Read the model definition and answer for the solid it produces. Units are mm, in the model's axes. A direction names the side the tool comes from. Give positions to 0.01 mm unless a question says otherwise; leave off trailing zeros. Loops run counter-clockwise (first coordinate to the right, second up) from the corner with the lowest first, then second, coordinate; pieces in that order, holes last.
(1) Find section B-B, the plane y = 40. Write down the section's boundary in (x, z), then the cut area to 3 significant figures.
(2) Each of these flat-tipped pins is pushed along its axis until it touches: P1, Ø19, axis at y = 73.5, z = -20, coming from the -X side; P2, Ø3, axis at x = 30, y = 67, coming from the +Z side; P3, Ø3, axis at x = 30.5, z = 5.5, coming from the +Y side. Where does it stop, or does it pass through?
(3) Which of the six approach directions +Z, -Z, +X, -X, +Y, -Y give full straight-line access (tool end or side, diameter ignored) to faces 4 (the face through (56, 12.5, -15)), 5 (the face through (3.89, 43.24, 5.27)), 6 (the face through (13.05, 23.01, 6.51))?
(4) Find section A-A, the plane x = 30. State how many separate pieces and enclosed holes the cut face has, then the cut area to 3 significant figures.
(5) Determine the mould class of faces 1 (the face through (30, 80, -3)), 2 (the face through (4, 4, -30)), 3 (the face through (3.5, 65, -2.5)) for opening direction Y: pulls with the +Y half, pulls with the -Y half, needs draft (parallel to the pull), parting line crosses it, or undercut.
(6) Find section D-D, the plane z = -17. Write down the section's boundary in (x, y).
(7) Straight lines are drawn through the part: probe 1 along Y at (x, z) = (56, -23); probe 2 along Z at (x, y) = (55.75, 5); probe 3 along Y at (x, z) = (52, -4.5). For each, find the intervals that lie inside material, in ascending order.
```python
from build123d import *

# Parameters (mm, degrees)
SKETCH1_W               = 60
SKETCH1_H               = 80
BOSS_EXTRUDE1_DEPTH     = 7
SKETCH2_W               = 7
SKETCH2_H               = 12.5
BOSS_EXTRUDE2_DEPTH     = 30
SKETCH3_R               = 2.6
CUT_EXTRUDE1_DEPTH      = 50
SKETCH4_R               = 25
CUT_EXTRUDE2_DEPTH      = 107.625512894
SKETCH6_R               = 2.1
CUT_EXTRUDE3_DEPTH      = 107.625512894
MIRROR2_COPY_1_SKETCH_W = 7
MIRROR2_COPY_1_SKETCH_H = 12.5
MIRROR2_COPY_1_DEPTH    = 30
MIRROR2_COPY_2_SKETCH_R = 2.6
MIRROR2_COPY_2_DEPTH    = 50
CHAMFER1_SIZE           = 5
CHAMFER2_SIZE           = 5
SKETCH9_W               = 46
SKETCH9_H               = 7.5
BOSS_EXTRUDE4_DEPTH     = 5
CHAMFER3_SIZE           = 5
SKETCH20_R              = 25
SKETCH20_R_2            = 23
BOSS_EXTRUDE5_DEPTH     = 1
CUT_EXTRUDE5_DEPTH      = 3.5


with BuildPart() as part:
    # Sketch1 → Boss-Extrude1 (new body)
    with BuildSketch(Plane.XY):
        with Locations((30, 40)):
            Rectangle(SKETCH1_W, SKETCH1_H)
    extrude(amount=BOSS_EXTRUDE1_DEPTH)

    # Sketch2 → Boss-Extrude2 (add)
    with BuildSketch(Plane(origin=(0, 0, 0), x_dir=(-1, 0, 0), z_dir=(0, 0, -1))):
        with Locations((-3.5, 73.75)):
            Rectangle(SKETCH2_W, SKETCH2_H)
    boss_extrude2 = extrude(amount=BOSS_EXTRUDE2_DEPTH)

    # Sketch3 → Cut-Extrude1 (cut)
    with BuildSketch(Plane.ZY):
        with Locations((-13, 75)):
            Circle(SKETCH3_R)
        with Locations((-23, 75)):
            Circle(SKETCH3_R)
    cut_extrude1 = extrude(amount=-CUT_EXTRUDE1_DEPTH, mode=Mode.SUBTRACT)

    # Sketch4 → Cut-Extrude2 (cut, through all)
    with BuildSketch(Plane.XY.offset(7)):
        with Locations((30, 40)):
            Circle(SKETCH4_R)
    extrude(amount=-CUT_EXTRUDE2_DEPTH, mode=Mode.SUBTRACT)

    # Sketch6 → Cut-Extrude3 (cut, through all)
    with BuildSketch(Plane.XY.offset(7)):
        with Locations((30, 67.5)):
            Circle(SKETCH6_R)
        with Locations((49.445436483, 59.445436483)):
            Circle(SKETCH6_R)
        with Locations((57.5, 40)):
            Circle(SKETCH6_R)
        with Locations((49.445436483, 20.554563517)):
            Circle(SKETCH6_R)
        with Locations((30, 12.5)):
            Circle(SKETCH6_R)
        with Locations((10.554563517, 20.554563517)):
            Circle(SKETCH6_R)
        with Locations((2.5, 40)):
            Circle(SKETCH6_R)
        with Locations((10.554563517, 59.445436483)):
            Circle(SKETCH6_R)
    extrude(amount=-CUT_EXTRUDE3_DEPTH, mode=Mode.SUBTRACT)

    # Mirror1: Boss-Extrude2, Cut-Extrude1 across plane
    add(boss_extrude2.mirror(Plane(origin=(0, 40, 0), x_dir=(0, 0, 1), z_dir=(0, -1, 0))))
    add(cut_extrude1.mirror(Plane(origin=(0, 40, 0), x_dir=(0, 0, 1), z_dir=(0, -1, 0))), mode=Mode.SUBTRACT)

    # Mirror2: Boss-Extrude2, Cut-Extrude1 across plane
    add(boss_extrude2.mirror(Plane(origin=(30, 0, 0), x_dir=(0, 0, 1), z_dir=(1, 0, 0))))
    add(cut_extrude1.mirror(Plane(origin=(30, 0, 0), x_dir=(0, 0, 1), z_dir=(1, 0, 0))), mode=Mode.SUBTRACT)

    # Mirror2 copy 1 sketch → Mirror2 copy 1 (add)
    with BuildSketch(Plane(origin=(60, 80, 0), x_dir=(1, 0, 0), z_dir=(0, 0, -1))):
        with Locations((-3.5, 73.75)):
            Rectangle(MIRROR2_COPY_1_SKETCH_W, MIRROR2_COPY_1_SKETCH_H)
    extrude(amount=MIRROR2_COPY_1_DEPTH)

    # Mirror2 copy 2 sketch → Mirror2 copy 2 (cut)
    with BuildSketch(Plane(origin=(60, 80, 0), x_dir=(0, 0, 1), z_dir=(1, 0, 0))):
        with Locations((-13, 75)):
            Circle(MIRROR2_COPY_2_SKETCH_R)
        with Locations((-23, 75)):
            Circle(MIRROR2_COPY_2_SKETCH_R)
    extrude(amount=-MIRROR2_COPY_2_DEPTH, mode=Mode.SUBTRACT)

    # Chamfer1
    chamfer1_edges = [part.edges().sort_by_distance(p)[0] for p in [
        (56.5, 67.5, 0),
        (56.5, 12.5, 0),
        (3.5, 67.5, 0),
        (3.5, 12.5, 0),
    ]]
    chamfer(chamfer1_edges, length=CHAMFER1_SIZE)

    # Chamfer2
    chamfer2_edges = [part.edges().sort_by_distance(p)[0] for p in [
        (56.5, 67.5, -30),
        (56.5, 12.5, -30),
        (3.5, 67.5, -30),
        (3.5, 12.5, -30),
    ]]
    chamfer(chamfer2_edges, length=CHAMFER2_SIZE)

    # Sketch9 → Boss-Extrude4 (add)
    with BuildSketch(Plane(origin=(0, 0, 0), x_dir=(-1, 0, 0), z_dir=(0, 0, -1))):
        with Locations((-30, 76.25)):
            Rectangle(SKETCH9_W, SKETCH9_H)
        with Locations((-30, 3.75)):
            Rectangle(SKETCH9_W, SKETCH9_H)
    extrude(amount=BOSS_EXTRUDE4_DEPTH)

    # Chamfer3
    chamfer3_edges = [part.edges().sort_by_distance(p)[0] for p in [
        (30, 80, 7),
        (30, 0, 7),
    ]]
    chamfer(chamfer3_edges, length=CHAMFER3_SIZE)

    # Sketch20 → Boss-Extrude5 (add)
    with BuildSketch(Plane.XY.offset(7)):
        with Locations((30, 40)):
            Circle(SKETCH20_R)
        with Locations((30, 40)):
            Circle(SKETCH20_R_2, mode=Mode.SUBTRACT)
    extrude(amount=-BOSS_EXTRUDE5_DEPTH)

    # Sketch21 → Cut-Extrude5 (cut)
    with BuildSketch(Plane.XY.offset(7)):
        Polygon((52.303174516, 56.587698449), (53.349179233, 60.4914412), (50.4914412, 63.349179233), (46.587698449, 62.303174516), (45.541693732, 58.399431765), (48.399431765, 55.541693732), align=None)
        Polygon((34.041451884, 67.5), (32.020725942, 71), (27.979274058, 71), (25.958548116, 67.5), (27.979274058, 64), (32.020725942, 64), align=None)
        Polygon((57.5, 35.958548116), (61, 37.979274058), (61, 42.020725942), (57.5, 44.041451884), (54, 42.020725942), (54, 37.979274058), align=None)
        Polygon((46.587698449, 17.696825484), (50.4914412, 16.650820767), (53.349179233, 19.5085588), (52.303174516, 23.412301551), (48.399431765, 24.458306268), (45.541693732, 21.600568235), align=None)
        Polygon((25.958548116, 12.5), (27.979274058, 9), (32.020725942, 9), (34.041451884, 12.5), (32.020725942, 16), (27.979274058, 16), align=None)
        Polygon((7.696825484, 23.412301551), (6.650820767, 19.5085588), (9.5085588, 16.650820767), (13.412301551, 17.696825484), (14.458306268, 21.600568235), (11.600568235, 24.458306268), align=None)
        Polygon((2.5, 44.041451884), (-1, 42.020725942), (-1, 37.979274058), (2.5, 35.958548116), (6, 37.979274058), (6, 42.020725942), align=None)
        Polygon((13.412301551, 62.303174516), (9.5085588, 63.349179233), (6.650820767, 60.4914412), (7.696825484, 56.587698449), (11.600568235, 55.541693732), (14.458306268, 58.399431765), align=None)
    extrude(amount=-CUT_EXTRUDE5_DEPTH, mode=Mode.SUBTRACT)


solid = part.part
```
Entries:
1. outline: (0, 0) - (0.4, 0) - (0.4, 3.5) - (0, 3.5) - close; (4.6, 0) - (5, 0) - (5, 3.5) - (4.6, 3.5) - close; (6, 6) - (7, 6) - (7, 7) - (6, 7) - close; (53, 6) - (54, 6) - (54, 7) - (53, 7) - close; (55, 0) - (55.4, 0) - (55.4, 3.5) - (55, 3.5) - close; (59.6, 0) - (60, 0) - (60, 3.5) - (59.6, 3.5) - close
1. area: 7.60 mm2
2. P1: stops at x = 0
2. P2: passes through
2. P3: stops at y = 78
3. face 4: -Z, +X, -X
3. face 5: +Z
3. face 6: +Z, -Z
4. separate pieces: 6
4. enclosed holes: 0
4. area: 191 mm2
5. face 1: pulls with the +Y half
5. face 2: needs draft
5. face 3: undercut
6. outline: (0, 0) - (7, 0) - (7, 12.5) - (0, 12.5) - close; (0, 67.5) - (7, 67.5) - (7, 80) - (0, 80) - close; (53, 0) - (60, 0) - (60, 12.5) - (53, 12.5) - close; (53, 67.5) - (60, 67.5) - (60, 80) - (53, 80) - close
7. probe 1: y = 0 to 2.4, 7.6 to 12.5, 67.5 to 72.4, 77.6 to 80
7. probe 2: z = -30 to -25.6, -20.4 to -15.6, -10.4 to 7
7. probe 3: y = 0 to 7.5, 72.5 to 80
